Input: part model. Units: mm. Frame: model coordinates. A direction names the side the tool comes from. Coordinates: 2 decimals unless noted, no trailing zeros. Write each loop counter-clockwise with the first axis right and the second up, starting at its lowest first coordinate (ties: lowest second). Pieces come first, ordered by that corner, then holes.
1) Section query A-A (z = 28.5). Output: boundary loops of the cut face in (x, y) (3 decimals).
2) Line query: L1, parallel to Z at x = 0, y = 24.5; L2, parallel to Y at x = -31.5, z = 3; L3, parallel to Y at x = 30, z = 19. Output: solid intervals per line, ascending.
3) Draft query along X for faces 3 (the flat face through (-19.904, 52.207, 16.762)), 4 (the cylindrical face through (-28.52, 24.04, 9.86)), 5 (the cylindrical face through (34.36, -32.87, 16.76)), 6 (the flat face through (-12, 6, 34)). Return one class per face: pulls with the +X half, pulls with the -X half, needs draft (parallel to the pull), parting line crosses it, or undercut.
4) Set-up query: faces 1 (the flat face through (-23.78, 35.06, 9.86)), 2 (the flat face through (3, 34, 0)). Return all of +Z, -Z, +X, -X, +Y, -Y with unobstructed straight access to the full face (end or side cutting, diameter ignored); none if empty.
5) Section query B-B (x = 31). State how many separate pieces and enclosed holes the cut face has, then the cut area to 3 significant figures.
6) Pin query (flat end, axial travel): pin 1 Ø4 at (x, y) = (10, 11) entering from -Z; pin 2 Ø1 at (x, z) = (-1.5, 27.5) entering from +Y; pin 3 Ø12 at (x, z) = (30.5, 11) entering from +Y. Return the tip coordinate at first contact, or that it passes through.
from build123d import *

# Parameters (mm, degrees)
SKETCH3_R                     = 50
SKETCH3_R_2                   = 2.75
EXTRUDE1_DEPTH                = 34
CUT_EXTRUDE2_DEPTH            = 20
EXTRUDE6_DEPTH                = 34
M16_75_16_75_DIAMETER_HOLE1_D = 16.75
CUT_EXTRUDE3_REACH            = 116.262
SKETCH22_R                    = 6.8


with BuildPart() as part:
    # Sketch3 → Extrude1 (new body)
    with BuildSketch(Plane.XY):
        Circle(SKETCH3_R)
        with Locations((31.819805153, -31.819805153)):
            Circle(SKETCH3_R_2, mode=Mode.SUBTRACT)
        with Locations((-31.819805153, -31.819805153)):
            Circle(SKETCH3_R_2, mode=Mode.SUBTRACT)
        with Locations((31.819805153, 31.819805153)):
            Circle(SKETCH3_R_2, mode=Mode.SUBTRACT)
        with Locations((-31.819805153, 31.819805153)):
            Circle(SKETCH3_R_2, mode=Mode.SUBTRACT)
    extrude(amount=EXTRUDE1_DEPTH)

    # Sketch3_6 → Cut-Extrude2 (cut)
    with BuildSketch(Plane.XY):
        with BuildLine():
            Line((-20.421328258, 43.144950309), (-27.237880936, 26.740610009))
            ThreePointArc((-27.237880936, 26.740610009), (-28.54324707, 23.999538948), (-30.118972052, 21.404439318))
            add(Edge.make_bspline(
                [(-8.411618966, 31.392589354), (-6.594986557, 31.927343906), (-4.727596656, 32.304011663), (-0.947579394, 32.726950043), (0.964989801, 32.773208373), (4.777108777, 32.531081057), (6.676598891, 32.242693441), (10.404207822, 31.337263886), (12.232267294, 30.720230446), (15.760360448, 29.173637758), (17.460336939, 28.244097303), (20.679062247, 26.098347596), (22.197757805, 24.882166939), (25.005835643, 22.198009273), (26.295170268, 20.730069861), (28.60307704, 17.585286262), (29.621608652, 15.90848759), (31.354425209, 12.395644964), (32.068678043, 10.559653108), (33.168512452, 6.783381836), (33.554071399, 4.84315955), (33.981977998, 0.91703866), (34.024313279, -1.068799499), (33.761644813, -5.025657895), (33.456639413, -6.996616206), (32.505786005, -10.863180522), (31.859947203, -12.758725015), (30.244434466, -16.415746217), (29.274780398, -18.177163724), (27.038718465, -21.510852538), (25.772340603, -23.083068793), (22.979235835, -25.988634722), (21.452548225, -27.321935222), (18.18350905, -29.706877352), (16.441204938, -30.758477245), (12.792592203, -32.545523582), (10.886337796, -33.28093707), (6.966927518, -34.410539179), (4.95383101, -34.804704707), (0.881572969, -35.237007362), (-1.17752584, -35.275132047), (-5.279057127, -34.991353155), (-7.321425423, -34.669448256), (-11.326780574, -33.672621975), (-13.289703752, -32.997710517), (-17.075395447, -31.312765708), (-18.898102754, -30.302753307), (-22.346412369, -27.975919739), (-23.971957836, -26.659129989), (-26.974594454, -23.756685335), (-28.351634915, -22.171071432), (-30.813133029, -18.777462502), (-31.89754775, -16.969516871), (-33.738297145, -13.184908034), (-34.494598024, -11.208301165), (-35.653409825, -7.145620969), (-36.055897198, -5.05960924), (-36.492023631, -0.841182208), (-36.525650191, 1.29116809), (-36.220191785, 5.537304064), (-35.881105833, 7.651023301), (-34.837758132, 11.795003117), (-34.13350703, 13.825197856), (-32.378618873, 17.739300975), (-31.328003859, 19.623146143), (-30.118972052, 21.404439318)],
                knots=[0, 0, 0, 0, 0.03125, 0.03125, 0.0625, 0.0625, 0.09375, 0.09375, 0.125, 0.125, 0.15625, 0.15625, 0.1875, 0.1875, 0.21875, 0.21875, 0.25, 0.25, 0.28125, 0.28125, 0.3125, 0.3125, 0.34375, 0.34375, 0.375, 0.375, 0.40625, 0.40625, 0.4375, 0.4375, 0.46875, 0.46875, 0.5, 0.5, 0.53125, 0.53125, 0.5625, 0.5625, 0.59375, 0.59375, 0.625, 0.625, 0.65625, 0.65625, 0.6875, 0.6875, 0.71875, 0.71875, 0.75, 0.75, 0.78125, 0.78125, 0.8125, 0.8125, 0.84375, 0.84375, 0.875, 0.875, 0.90625, 0.90625, 0.9375, 0.9375, 0.96875, 0.96875, 1, 1, 1, 1], degree=3))
            Line((-8.411618966, 31.392589354), (-6.015539335, 37.158862647))
            Line((-6.015539335, 37.158862647), (-20.421328258, 43.144950309))
        make_face()
    extrude(amount=CUT_EXTRUDE2_DEPTH, mode=Mode.SUBTRACT)

    # Sketch3_7 → Extrude6 (add)
    with BuildSketch(Plane.XY):
        with BuildLine():
            ThreePointArc((-23.191672282, 44.296121013), (-21.196140075, 45.284916318), (-19.158555872, 46.183868795))
            ThreePointArc((-19.158555872, 46.183868795), (-10.101449269, 48.968977145), (-0.681547061, 49.99535472))
            ThreePointArc((-0.681547061, 49.99535472), (4.254411372, 49.818671037), (9.148855424, 49.155858699))
            Line((9.148855424, 49.155858699), (-16.707688798, 59.900118605))
            Line((-16.707688798, 59.900118605), (-23.191672282, 44.296121013))
        make_face()
    extrude(amount=EXTRUDE6_DEPTH)

    # M16.75 _16.75_ Diameter Hole1 (through all)
    with Locations(Plane.XY.offset(34)):
        with Locations((0, 0)):
            Hole(M16_75_16_75_DIAMETER_HOLE1_D / 2)

    # Sketch22 → Cut-Extrude3 (cut, up to next)
    with BuildSketch(Plane(origin=(18.765429823, 45.159850034, 0), x_dir=(-0.923448008, 0.383723568, 0), z_dir=(0.383723568, 0.923448008, 0)), mode=Mode.PRIVATE) as cut_extrude3_sk1:
        with Locations((27.613769175, 12)):
            Circle(SKETCH22_R)
    cut_extrude3_tool1 = extrude(cut_extrude3_sk1.sketch, amount=-CUT_EXTRUDE3_REACH, mode=Mode.PRIVATE) & part.part
    add(cut_extrude3_tool1.solids().sort_by_distance((-6.73445, 55.755904, 12))[0], mode=Mode.SUBTRACT)


solid = part.part
Answer:
1. outline: (-23.192, 44.296) arc R50 ccw (long way) to (9.149, 49.156) - (-16.708, 59.9) - close; hole circle Ø5.5 at (-31.82, -31.82); hole circle Ø5.5 at (-31.82, 31.82); hole circle Ø16.75 at (0, 0); hole circle Ø5.5 at (31.82, -31.82); hole circle Ø5.5 at (31.82, 31.82)
2. L1: z = 20 to 34
2. L2: y = -38.83 to -34.55, -29.09 to -17.54, 19.21 to 29.09, 34.55 to 38.83
2. L3: y = -40 to -33.88, -29.76 to -16.76, 15.1 to 29.76, 33.88 to 40
3. face 3: pulls with the -X half
3. face 4: undercut
3. face 5: undercut
3. face 6: needs draft
4. face 1: -Z
4. face 2: -Z, +X, -X, +Y, -Y
5. separate pieces: 3
5. enclosed holes: 0
5. area: 1,760 mm2
6. pin 1: stops at z = 20
6. pin 2: stops at y = 53.79
6. pin 3: stops at y = 43.59
